Could you check a few things on this model? Use its own coordinates, in mm. Coordinates: 2 decimals unless noted, no trailing zeros. Order: outer loops, then holes, each group sorted by start corner. A loop starts at its lowest first (then second) coordinate and runs counter-clockwise, first axis right, second up. Notation, with made-up numbers: (56, 71) - (82, 71) arc R20 cw to (82, 78) - close; hole circle Ø8 at (36.25, 52.25). An arc over 180 degrees is marked (long way). One line per item, written item: value.
from build123d import *

# Parameters (mm, degrees)
SKETCH_1_W          = 20
SKETCH_1_H          = 68
SKETCH_1_R          = 2.2
EXTRUDE_1_DEPTH     = 5
FILLET_1_R          = 5
SKETCH_2_R          = 2
CUT_EXTRUDE_1_DEPTH = 10


with BuildPart() as part:
    # ｽｹｯﾁ1 → ﾎﾞｽ - 押し出し1 (new body)
    with BuildSketch(Plane.XY):
        with Locations((10, 34)):
            Rectangle(SKETCH_1_W, SKETCH_1_H)
        with Locations((10, 10)):
            Circle(SKETCH_1_R, mode=Mode.SUBTRACT)
    extrude(amount=EXTRUDE_1_DEPTH)

    # ﾌｨﾚｯﾄ1
    fillet_1_edges = [part.edges().sort_by_distance(p)[0] for p in [
        (20, 0, 2.5),
        (0, 0, 2.5),
    ]]
    fillet(fillet_1_edges, radius=FILLET_1_R)

    # ｽｹｯﾁ2 → ｶｯﾄ - 押し出し1 (cut)
    with BuildSketch(Plane(origin=(0, 68, 0), x_dir=(1, 0, 0), z_dir=(0, 1, 0))):
        with Locations(Location((10, -2.5, 0), (0, 0, 270))):
            Circle(SKETCH_2_R)
    extrude(amount=-CUT_EXTRUDE_1_DEPTH, mode=Mode.SUBTRACT)


solid = part.part
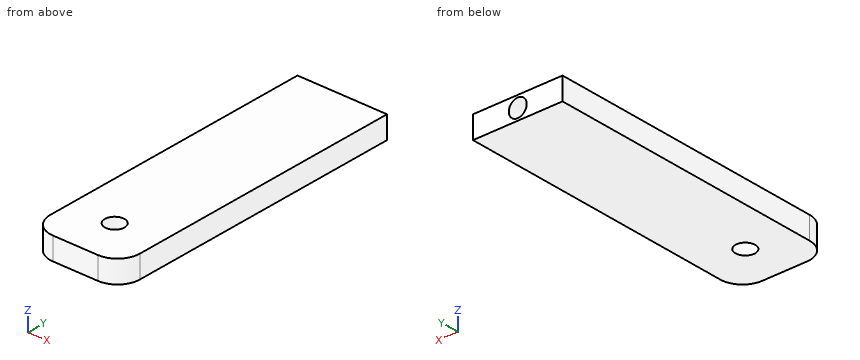
Item 1: I want a section at C-C on z = 2.5. Please give me the cut outline in (x, y), then the cut area to 3 significant figures.
Conclusion:
outline: (0, 5) arc R5 ccw to (5, 0) - (15, 0) arc R5 ccw to (20, 5) - (20, 68) - (12, 68) - (12, 58) - (8, 58) - (8, 68) - (0, 68) - close; hole circle Ø4.4 at (10, 10)
area: 1,290 mm²
Item 2: I want a section at B-B on y = 10. Please give me the cut outline in (x, z).
Conclusion:
outline: (0, 0) - (7.8, 0) - (7.8, 5) - (0, 5) - close; (12.2, 0) - (20, 0) - (20, 5) - (12.2, 5) - close
Item 3: I'm going to push a flat-ended pin straight in: pin 1 Ø2 at (x, z) = (9.5, 2) entering from +Y. Where does the tip first touch, or does it pass through?
Conclusion:
pin 1: y = 58
Item 4: I want a section at A-A on x = 10. Please give me the cut outline in (y, z), then the cut area to 3 significant figures.
Conclusion:
outline: (0, 0) - (7.8, 0) - (7.8, 5) - (0, 5) - close; (12.2, 0) - (68, 0) - (68, 0.5) - (58, 0.5) - (58, 4.5) - (68, 4.5) - (68, 5) - (12.2, 5) - close
area: 278 mm²
Item 5: If I drill on probe 1 along Y at (x, z) = (10, 1.4); probe 2 along X at (y, z) = (64, 2.5); probe 3 along X at (y, z) = (64, 3.2), over which ranges is the centre line in solid material (lowest first)?
Conclusion:
probe 1: 0 to 7.8, 12.2 to 58
probe 2: 0 to 8, 12 to 20
probe 3: 0 to 8.13, 11.87 to 20
Item 6: I want a section at D-D on x = 1.5. Please give me the cut outline in (y, z).
Conclusion:
outline: (1.43, 0) - (68, 0) - (68, 5) - (1.43, 5) - close
